Autodesk Inventor part; units mm, degrees
ref_plane "YZ Plane" through (0, 0, 0) normal (1, 0, 0) x (0, 1, 0)
ref_plane "XZ Plane" through (0, 0, 0) normal (0, 1, 0) x (-1, 0, 0)
ref_plane "XY Plane" through (0, 0, 0) normal (0, 0, 1) x (1, 0, 0)
sketch "Sketch1" plane through (0, 0, 0) normal (0, 1, 0) x (-1, 0, 0)
  line L0 (0, 0) -> (80, 0)
  line L1 (80, 0) -> (80, -14)
  line L2 (80, -14) -> (0, -14)
  line L3 (0, -14) -> (0, 0)
  line L4 (80, -2) -> (83, -2)
  line L5 (83, -2) -> (83, -12)
  line L6 (83, -12) -> (80, -12)
  line L7 (40, -14) -> (40, 0) construction
  line L8 (0, -2) -> (-3, -2)
  line L9 (-3, -2) -> (-3, -12)
  line L10 (-3, -12) -> (0, -12)
  dimension "d0" = 14
  dimension "d1" = 80
  dimension "d2" = 2
  dimension "d3" = 10
  dimension "d4" = 3
extrude "Extrusion1" add sketch "Sketch1" along normal blind 3
properties part number "soporte_base_parqueo"
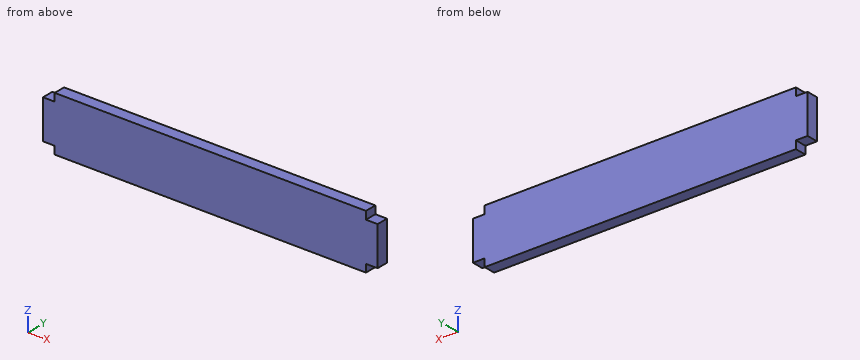
Verification items for the finished model (mm, model axes). Coordinates: 2 decimals unless noted, no trailing zeros. Loops run counter-clockwise (first coordinate to the right, second up) from the corner with the lowest first, then second, coordinate; pieces in that order, holes last. Notation, with made-up numbers: (-8, 15) -> (42, 15) arc R8 ccw to (42, 26) -> close; hole circle Ø7 at (81, -8.75). An arc over 180 degrees is marked (long way). Answer in a Markdown table with one row per item.
1) Depth check by flat-ended pin: P1, Ø1.6, axis at y = 1.5, z = -0.5, coming from the +X side; P2, Ø1.5, axis at x = -81, y = 1.5, coming from the -Z side; P3, Ø0.6, axis at y = 1, z = -1.5, coming from the -X side. Enter the tip coordinate at first touch or a pass-through.
The answers:
| item | result |
|---|---|
| P1 | stops at x = 0 |
| P2 | stops at z = -12 |
| P3 | stops at x = -80 |
2) Section check A-A (y = 1.05). Record the cut outline in (x, z).
The answers:
| item | result |
|---|---|
| outline | (-83, -12) -> (-80, -12) -> (-80, -14) -> (0, -14) -> (0, -12) -> (3, -12) -> (3, -2) -> (0, -2) -> (0, 0) -> (-80, 0) -> (-80, -2) -> (-83, -2) -> close |
3) Scan line: line 1 along X through (y, z) = (1.65, -12.25). Record every from-to range of solid material in increasing order. Write a range as from..to.
The answers:
| item | result |
|---|---|
| line 1 | x = -80..0 |
